Check sheet for the modelled part. Datum: model origin and axes. Units: mm. Face numbers are marked on the shaded views. A direction names the side the tool comes from. Round coordinates to 2 decimals unless told otherwise and drop trailing zeros. Order: outer loops, then holes, each group sorted by start corner. A loop starts at its lowest first (then second) coordinate and runs counter-clockwise, first axis right, second up. Notation, with made-up numbers: (11.25, 71.5) -> (44.25, 71.5) arc R28 ccw to (44.25, 105.5) -> close; hole circle Ø2 at (65.25, 60). An arc over 180 degrees is marked (long way). Answer in a Markdown table with one row per item.
```python
from build123d import *

# Parameters (mm, degrees)
F0_R     = 2.25
F0_R_2   = 1.55
F1_DEPTH = 15
F3_DEPTH = 6.501
F4_R     = 0.5


with BuildPart() as f1:
    # F0 (on Front) → F1 (new body)
    with BuildSketch(Plane.XZ):
        with BuildLine():
            ThreePointArc((-5.75, -3.25), (-3.451903, -2.298097), (-2.5, 0))
            ThreePointArc((-2.5, 0), (-3.451903, 2.298097), (-5.75, 3.25))
            ThreePointArc((-5.75, 3.25), (-9, 0), (-5.75, -3.25))
        make_face()
        with Locations((-5.75, 0)):
            Circle(F0_R, mode=Mode.SUBTRACT)
        with BuildLine():
            ThreePointArc((9, 0), (8.048097, 2.298097), (5.75, 3.25))
            ThreePointArc((5.75, 3.25), (2.5, 0), (5.75, -3.25))
            ThreePointArc((5.75, -3.25), (8.048097, -2.298097), (9, 0))
        make_face()
        with Locations((5.75, 0)):
            Circle(F0_R, mode=Mode.SUBTRACT)
        with BuildLine():
            ThreePointArc((-5.75, 3.25), (-3.451903, 2.298097), (-2.5, 0))
            ThreePointArc((-2.5, 0), (-3.451903, -2.298097), (-5.75, -3.25))
            Line((-5.75, -3.25), (5.75, -3.25))
            ThreePointArc((5.75, -3.25), (2.5, 0), (5.75, 3.25))
            Line((5.75, 3.25), (-5.75, 3.25))
        make_face()
        Circle(F0_R_2, mode=Mode.SUBTRACT)
    extrude(amount=F1_DEPTH)

    # F2 (on face) → F3 (cut, through all)
    with BuildSketch(Plane.XY.offset(3.25)):
        with BuildLine():
            ThreePointArc((-1, -12.5), (0, -13.5), (1, -12.5))
            ThreePointArc((1, -12.5), (0, -11.5), (-1, -12.5))
        make_face()
        with BuildLine():
            ThreePointArc((-1, -12.5), (0, -11.5), (1, -12.5))
            Line((1, -12.5), (1, -7.5))
            Line((1, -7.5), (1, -2.5))
            ThreePointArc((1, -2.5), (0, -3.5), (-1, -2.5))
            Line((-1, -2.5), (-1, -7.5))
            Line((-1, -7.5), (-1, -12.5))
        make_face()
        with BuildLine():
            ThreePointArc((-1, -2.5), (0, -3.5), (1, -2.5))
            ThreePointArc((1, -2.5), (0, -1.5), (-1, -2.5))
        make_face()
    extrude(amount=-F3_DEPTH, mode=Mode.SUBTRACT)

    # F4
    f4_edges = [f1.edges().sort_by_distance(p)[0] for p in [
        (0, 0, 3.25),
        (0, -15, 3.25),
    ]]
    fillet(f4_edges, radius=F4_R)


solid = f1.part
```
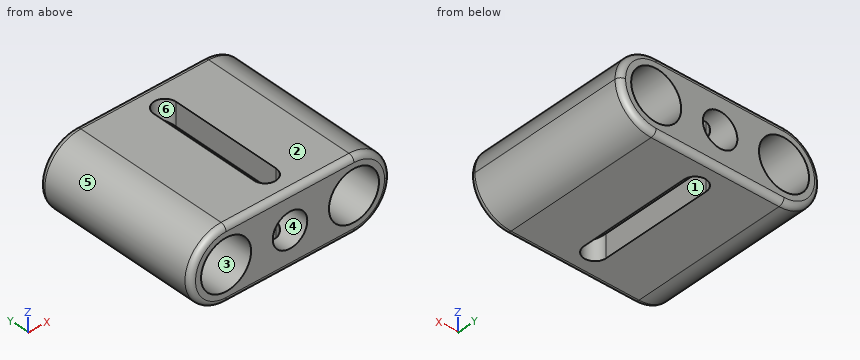
(1) Section check B-B on x = 0. Record the boundary of the cut face in (y, z).
Solutions:
| item | result |
|---|---|
| outline | (-15, -2.75) arc R0.5 ccw to (-14.5, -3.25) -> (-13.5, -3.25) -> (-13.5, -1.55) -> (-15, -1.55) -> close; (-15, 1.55) -> (-13.5, 1.55) -> (-13.5, 3.25) -> (-14.5, 3.25) arc R0.5 ccw to (-15, 2.75) -> close; (-1.5, -3.25) -> (-0.5, -3.25) arc R0.5 ccw to (0, -2.75) -> (0, -1.55) -> (-1.5, -1.55) -> close; (-1.5, 1.55) -> (0, 1.55) -> (0, 2.75) arc R0.5 ccw to (-0.5, 3.25) -> (-1.5, 3.25) -> close |
(2) Section check C-C on y = -0.75. Record the boundary of the cut face in (x, z).
Solutions:
| item | result |
|---|---|
| outline | (-5.75, -3.25) -> (5.75, -3.25) arc R3.25 ccw to (5.75, 3.25) -> (-5.75, 3.25) arc R3.25 ccw to start; hole circle Ø4.5 at (-5.75, 0); hole circle Ø3.1 at (0, 0); hole circle Ø4.5 at (5.75, 0) |
(3) Draft check along Z on the marked faces 3, 4, 5 and 6. Enter one of: pulls with the +Z half, pulls with the -Z half, needs draft (parallel to the pull), parting line crosses it, or undercut.
Solutions:
| item | result |
|---|---|
| face 3 | undercut |
| face 4 | undercut |
| face 5 | parting line crosses it |
| face 6 | needs draft |
(4) Section check A-A on y = -7.75. Record the boundary of the cut face in (x, z).
Solutions:
| item | result |
|---|---|
| outline | (-5.75, -3.25) -> (-1, -3.25) -> (-1, -1.18) arc R1.55 cw to (-1, 1.18) -> (-1, 3.25) -> (-5.75, 3.25) arc R3.25 ccw to start; (1, -3.25) -> (5.75, -3.25) arc R3.25 ccw to (5.75, 3.25) -> (1, 3.25) -> (1, 1.18) arc R1.55 cw to (1, -1.18) -> close; hole circle Ø4.5 at (-5.75, 0); hole circle Ø4.5 at (5.75, 0) |
(5) Scan lines: probe 1 along Z at (x, y) = (-5.75, -3.75); probe 2 along X at (y, z) = (-5, 1.75); probe 3 along X at (y, z) = (-7, 0.75). Record each from-to range of solid material in increasing order. Write a range as from..to.
Solutions:
| item | result |
|---|---|
| probe 1 | -3.25..-2.25, 2.25..3.25 |
| probe 2 | -8.49..-7.16, -4.34..-1, 1..4.34, 7.16..8.49 |
| probe 3 | -8.91..-7.87, -3.63..-1.36, 1.36..3.63, 7.87..8.91 |
(6) Section check D-D on x = 5.25. Record the boundary of the cut face in (y, z), plus the area to 3 significant figures.
Solutions:
| item | result |
|---|---|
| outline | (-15, -2.75) arc R0.5 ccw to (-14.5, -3.25) -> (-0.5, -3.25) arc R0.5 ccw to (0, -2.75) -> (0, -2.19) -> (-15, -2.19) -> close; (-15, 2.19) -> (0, 2.19) -> (0, 2.75) arc R0.5 ccw to (-0.5, 3.25) -> (-14.5, 3.25) arc R0.5 ccw to (-15, 2.75) -> close |
| area | 31.5 mm^2 |
(7) Depth check by flat-ended pin: pin 1 Ø1.7 at (y, z) = (-7, 2) entering from -X; pin 2 Ø2.5 at (y, z) = (-9.5, 2.5) entering from +X; pin 3 Ø1.7 at (y, z) = (-6, -2.5) entering from -X. Enter the tip coordinate at first touch or a pass-through.
Solutions:
| item | result |
|---|---|
| pin 1 | x = -8.79 |
| pin 2 | x = 8.75 |
| pin 3 | x = -8.55 |
(8) Tool access check on the marked faces 1 and 2. Record the directions out of +Z, -Z, +X, -X, +Y, -Y that give a thin tool (end or side, any length) a straight path to the whole face; none if there is none.
Solutions:
| item | result |
|---|---|
| face 1 | +Z, -Z |
| face 2 | +Z, +X, -X, +Y, -Y |
